Autodesk Inventor part; units mm, degrees
ref_plane "YZ Plane" through (0, 0, 0) normal (1, 0, 0) x (0, 1, 0)
ref_plane "XZ Plane" through (0, 0, 0) normal (0, 1, 0) x (-1, 0, 0)
ref_plane "XY Plane" through (0, 0, 0) normal (0, 0, 1) x (1, 0, 0)
sketch "Sketch1" plane through (0, 0, 0) normal (0, 1, 0) x (-1, 0, 0)
  line L0 (4, 0) -> (-4, 0)
  line L1 (4, 0) -> (4, 12)
  line L2 (-4, 0) -> (-4, 12)
  arc A0 (4, 17.3329) -> (-4, 17.3329) centre (0, 17.3329) ccw
  line L3 (4, 17.3329) -> (4, 12)
  line L4 (-4, 17.3329) -> (-4, 12)
  circle A1 centre (0, 17.3329) radius 1.65
  point P0 (0, 0)
  point P1 (0, 0)
  dimension "d0" = 8
  dimension "d1" = 12
  dimension "d9" = 8
  dimension "d12" = 3.3
extrude "Extrusion1" add sketch "Sketch1" along normal blind 3
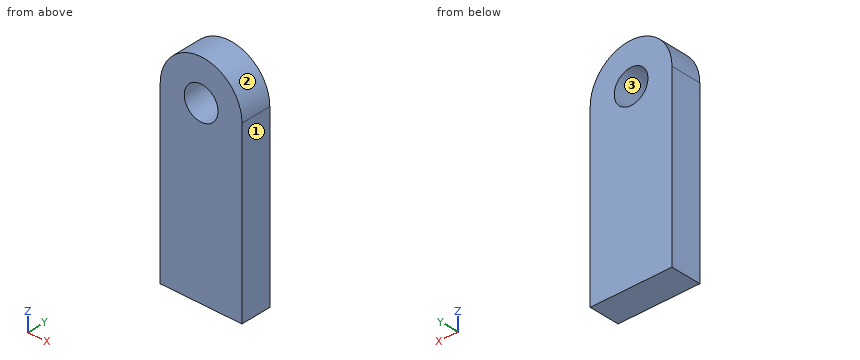
Design review of the part built by this model. Coordinates are the model's own, in mm. Face numbers are marked on the shaded views. Round coordinates to 2 decimals unless told otherwise and drop trailing zeros. Write each loop counter-clockwise with the first axis right and the second up, starting at its lowest first coordinate (ties: lowest second). Pieces come first, ordered by that corner, then holes.
Item 1: For probe 1 along Z at (x, y) = (0, 1); probe 2 along Z at (x, y) = (1.5, 0.3); probe 3 along X at (y, z) = (2.75, 17), list the stretches that pass through material, from the lowest coordinate up.
Item 2: We need section A-A on x = 0. Write out the cut boundary in (y, z).
Item 3: We need section B-B on y = 1.1. Write out the cut boundary in (x, z), and give its area (3 significant figures).
Item 4: The part is to be moulded in two halves that separate along X. For the marked faces 1, 2 and 3, say which applies: +X half, -X half, draft (parallel to the pull), parting line (faces both ways), or undercut.
Returned:
1. probe 1: z = 0 to 15.68, 18.98 to 21.33
1. probe 2: z = 0 to 16.65, 18.02 to 21.04
1. probe 3: x = -4 to -1.62, 1.62 to 4
2. outline: (0, 0) - (3, 0) - (3, 15.68) - (0, 15.68) - close; (0, 18.98) - (3, 18.98) - (3, 21.33) - (0, 21.33) - close
3. outline: (-4, 0) - (4, 0) - (4, 17.33) arc R4 ccw to (-4, 17.33) - close; hole circle Ø3.3 at (0, 17.33)
3. area: 155 mm2
4. face 1: +X half
4. face 2: parting line
4. face 3: undercut
